Here's the drawing with two shaded views (mm, measured from the low corner). I have some questions. A direction names the side the tool comes from. Round coordinates to 2 decimals unless told otherwise and drop trailing zeros. Loops run counter-clockwise (first coordinate to the right, second up) from the corner with the lowest first, then second, coordinate; pieces in that order, holes last. Notation, with made-up numbers: (78.5, -1.75) - (95.5, -1.75) arc R30 ccw to (95.5, 30.25) - close; hole circle Ø2 at (18.25, -21). An arc over 180 degrees is marked (long way). Use one line per item in the form item = value.
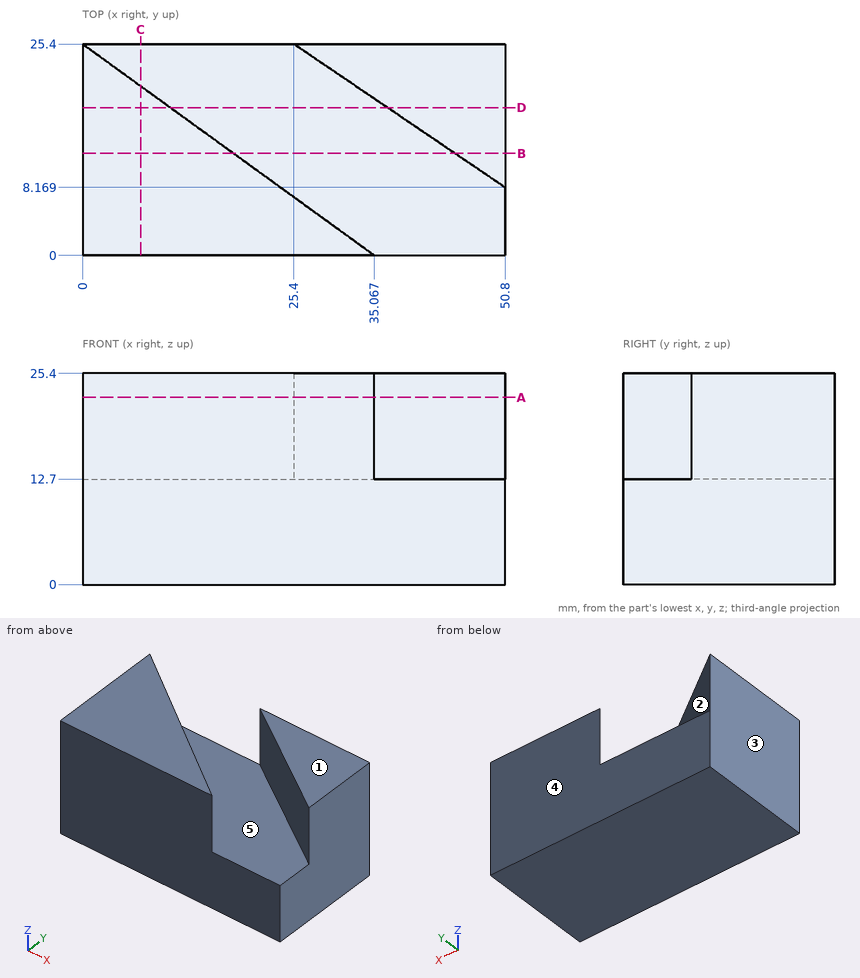
1. If we section it at D-D, the plane y = 17.75: Write out the boundary of the cut face in (x, z).
Solution:
outline = (0, 0) - (50.8, 0) - (50.8, 25.4) - (36.68, 25.4) - (36.68, 12.7) - (10.56, 12.7) - (10.56, 25.4) - (0, 25.4) - close
2. On a 3-axis mill with a long thin cutter (end or side, diameter ignored), from which of +Z, -Z, +X, -X, +Y, -Y can I reach the whole of each face in a straight line? I mean the marked faces 4 and 5. Say none if no direction works.
Solution:
face_4 = +Z, -Z, +X, -X, +Y
face_5 = +Z
3. We'd pull the mould along X, two halves only. Please class the marked faces 1, 2 and 3: +X half, -X half, draft (parallel to the pull), parting line (faces both ways), or undercut.
Solution:
face_1 = draft
face_2 = undercut
face_3 = -X half
4. If we section it at C-C, the plane x = 7: Write out the boundary of the cut face in (y, z), plus the area to 3 significant figures.
Solution:
outline = (0, 0) - (25.4, 0) - (25.4, 12.7) - (20.33, 12.7) - (20.33, 25.4) - (0, 25.4) - close
area = 581 mm^2
5. For P1, Ø7.5, axis at x = 15.5, y = 17, coming from the +Z side; P2, Ø5, axis at x = 22.5, z = 18.5, coming from the +Y side; P3, Ø4, axis at x = 6, z = 16, coming from the +Y side, each with a flat end and sliding along its axis, tell me the tip position at first contact or that it passes through.
Solution:
P1 = 25.4
P2 = 10.91
P3 = 22.5
6. If we section it at A-A, the plane z = 22.5: Write out the boundary of the cut face in (x, y), plus the area to 3 significant figures.
Solution:
outline = (0, 0) - (35.07, 0) - (0, 25.4) - close; (25.4, 25.4) - (50.8, 8.17) - (50.8, 25.4) - close
area = 664 mm^2
7. If we section it at B-B, the plane y = 12.25: Write out the boundary of the cut face in (x, z) (1 decimal).
Solution:
outline = (0, 0) - (50.8, 0) - (50.8, 25.4) - (44.8, 25.4) - (44.8, 12.7) - (18.2, 12.7) - (18.2, 25.4) - (0, 25.4) - close
8. Please list where these lines run through material, in increasing order: line 1 along Z through (x, y) = (28, 16.75); line 2 along X through (y, z) = (9, 13.5) (1 decimal); line 3 along X through (y, z) = (21.25, 22.25) (1 decimal).
Solution:
line_1 = 0 to 12.7
line_2 = 0 to 22.6, 49.6 to 50.8
line_3 = 0 to 5.7, 31.5 to 50.8
